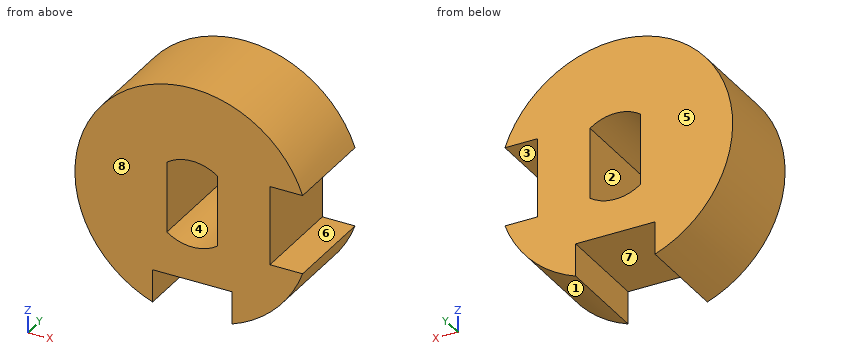
from build123d import *

# Parameters (mm, degrees)
BOSS_EXTRUDE1_DEPTH = 6


with BuildPart() as part:
    # Sketch1 → Boss-Extrude1 (new body)
    with BuildSketch(Plane(origin=(0, 0, 0), x_dir=(1, 0, 0), z_dir=(0, 1, 0))):
        with BuildLine():
            Line((4.9, -2.5), (4.9, 2.5))
            Line((4.9, 2.5), (6.96491206, 2.5))
            ThreePointArc((6.96491206, 2.5), (5.232590181, 5.232590181), (2.5, 6.96491206))
            Line((2.5, 6.96491206), (2.5, 4.9))
            Line((2.5, 4.9), (-2.5, 4.9))
            Line((-2.5, 4.9), (-2.5, 6.96491206))
            ThreePointArc((-2.5, 6.96491206), (-5.232590181, -5.232590181), (6.96491206, -2.5))
            Line((6.96491206, -2.5), (4.9, -2.5))
        make_face()
        with BuildLine():
            Line((-1.6, -2.236626925), (-1.6, 2.236626925))
            ThreePointArc((-1.6, 2.236626925), (0, 2.75), (1.6, 2.236626925))
            Line((1.6, 2.236626925), (1.6, -2.236626925))
            ThreePointArc((1.6, -2.236626925), (0, -2.75), (-1.6, -2.236626925))
        make_face(mode=Mode.SUBTRACT)
    extrude(amount=BOSS_EXTRUDE1_DEPTH)


solid = part.part
Read the model definition and answer for the solid it produces. Units are mm, in the model's axes. Face numbers are marked on the shaded views. A direction names the side the tool comes from. Coordinates: 2 decimals unless noted, no trailing zeros. Write each loop counter-clockwise with the first axis right and the second up, starting at its lowest first coordinate (ties: lowest second). Pieces come first, ordered by that corner, then holes. Notation, with made-up numbers: (55.25, 40.25) - (86.25, 40.25) arc R36 cw to (86.25, 76.25) - close; hole circle Ø10 at (78, 83). An arc over 180 degrees is marked (long way). One line per question, with ' | ' between items.
Q1. For the marked faces 4, 5, 6, 7 and 8, determine the directions among +Z, -Z, +X, -X, +Y, -Y from which every point of the face is accessible in a straight line to the end or side of a thin tool.
Result set:
face 4: +Y, -Y | face 5: +Z, -Z, +X, -X, +Y | face 6: +X, +Y, -Y | face 7: -Z, +Y, -Y | face 8: +Z, -Z, +X, -X, -Y
Q2. Determine the mould class of the marked faces 1, 2 and 3 for opening direction X: +X half, -X half, draft (parallel to the pull), parting line (faces both ways), or undercut.
Result set:
face 1: +X half | face 2: undercut | face 3: draft
Q3. Each of these flat-tipped pins is pushed along its axis until it touches: P1, Ø1.5, axis at x = -0.5, y = 2.5, coming from the -Z side; P2, Ø1.7, axis at x = 6, y = 3, coming from the +Z side; P3, Ø2, axis at y = 2, z = 0.5, coming from the +X side. Where does it stop, or does it pass through?
Result set:
P1: z = -4.9 | P2: z = 5.31 | P3: x = 4.9
Q4. Find section A-A, the plane y = 0.45. Write down the section's boundary in (x, z), plus the area to 3 significant figures.
Result set:
outline: (-2.5, -6.96) - (-2.5, -4.9) - (2.5, -4.9) - (2.5, -6.96) arc R7.4 ccw to (6.96, -2.5) - (4.9, -2.5) - (4.9, 2.5) - (6.96, 2.5) arc R7.4 ccw (long way) to start; hole (-1.6, -2.24) arc R2.75 ccw to (1.6, -2.24) - (1.6, 2.24) arc R2.75 ccw to (-1.6, 2.24) - close | area: 132 mm^2
Q5. Consider L1, parallel to X at y = 4.8, z = 0.75; L2, parallel to Z at x = -2.75, y = 2.85; L3, parallel to Z at x = -3.5, y = 2.55. Determine where each line is inside the solid, lowest interval first. Write a range as [from, to].
Result set:
L1: [-7.36, -1.6], [1.6, 4.9] | L2: [-6.87, 6.87] | L3: [-6.52, 6.52]
Q6. Find section C-C, the plane z = 0. Write down the section's boundary in (x, y), plus the area to 3 significant figures.
Result set:
outline: (-7.4, 0) - (-1.6, 0) - (-1.6, 6) - (-7.4, 6) - close; (1.6, 0) - (4.9, 0) - (4.9, 6) - (1.6, 6) - close | area: 54.6 mm^2
Q7. Find section B-B, the plane x = 0. Write down the section's boundary in (y, z), plus the area to 3 significant figures.
Result set:
outline: (0, -4.9) - (6, -4.9) - (6, -2.75) - (0, -2.75) - close; (0, 2.75) - (6, 2.75) - (6, 7.4) - (0, 7.4) - close | area: 40.8 mm^2
Q8. Find section D-D, the plane x = -4.75. Write down the section's boundary in (y, z).
Result set:
outline: (0, -5.67) - (6, -5.67) - (6, 5.67) - (0, 5.67) - close
